```python
from build123d import *

# Parameters (mm, degrees)
SKETCH1_W           = 3
SKETCH1_H           = 6
SKETCH1_W_2         = 16
SKETCH1_H_2         = 3
BOSS_EXTRUDE1_DEPTH = 3


with BuildPart() as part:
    # Sketch1 → Boss-Extrude1 (new body)
    with BuildSketch(Plane(origin=(0, 0, 0), x_dir=(1, 0, 0), z_dir=(0, 1, 0))):
        Polygon((60.5, 0), (60.5, 48), (36, 48), (20, 48), (0, 48), (0, 41), (0, 35), (0, 13), (0, 7), (0, 0), (20, 0), (36, 0), align=None)
        Polygon((85, 48), (60.5, 48), (60.5, 0), (85, 0), (101, 0), (121, 0), (121, 7), (121, 13), (121, 35), (121, 41), (121, 48), (101, 48), align=None)
        with Locations((-1.5, 10)):
            Rectangle(SKETCH1_W, SKETCH1_H)
        with Locations((28, -1.5)):
            Rectangle(SKETCH1_W_2, SKETCH1_H_2)
        with Locations((93, -1.5)):
            Rectangle(SKETCH1_W_2, SKETCH1_H_2)
        with Locations((122.5, 38)):
            Rectangle(SKETCH1_W, SKETCH1_H)
        with Locations((122.5, 10)):
            Rectangle(SKETCH1_W, SKETCH1_H)
        with Locations((-1.5, 38)):
            Rectangle(SKETCH1_W, SKETCH1_H)
        with Locations((28, 49.5)):
            Rectangle(SKETCH1_W_2, SKETCH1_H_2)
        with Locations((93, 49.5)):
            Rectangle(SKETCH1_W_2, SKETCH1_H_2)
    extrude(amount=BOSS_EXTRUDE1_DEPTH)


solid = part.part
```
Can you work these out from the model? Positions are in its coordinate system, mm. A direction names the side the tool comes from. Coordinates: 2 decimals unless noted, no trailing zeros. Write each loop counter-clockwise with the first axis right and the second up, starting at its lowest first coordinate (ties: lowest second). Pieces come first, ordered by that corner, then holes. Notation, with made-up numbers: (11.25, -8.75) - (55.25, -8.75) arc R15 ccw to (55.25, 6.25) - close; hole circle Ø2 at (5.5, 62.5). An arc over 180 degrees is marked (long way). Return JSON: item names as keys, results as strings.
Q1. Thinking about a two-plate mould opening in X: for faces 6 (the flat face through (28, 1, 3)), 7 (the flat face through (61, 1, -48)), 8 (the flat face through (101, 1, 2)), which applies, +X half, -X half, draft (parallel to the pull), parting line (faces both ways), or undercut?
Computed values:
{"face 6": "draft", "face 7": "undercut", "face 8": "+X half"}
Q2. On a 3-axis mill with a long thin cutter (end or side, diameter ignored), from which of +Z, -Z, +X, -X, +Y, -Y can I reach the whole of each face in a straight line? I mean faces 1 (the flat face through (10, 1, 0)), 2 (the flat face through (121, 1, -3)), 3 (the flat face through (60, 1, 0)), 4 (the flat face through (121, 1, -24)), 5 (the flat face through (36, 1, -49)). Say none if no direction works.
Computed values:
{"face 1": "+Z, -X, +Y, -Y", "face 2": "+Z, +X, +Y, -Y", "face 3": "+Z, +Y, -Y", "face 4": "+X, +Y, -Y", "face 5": "-Z, +Y, -Y"}
Q3. If we section it at A-A (x = 113.5): Please give me the cut outline in (y, z).
Computed values:
{"outline": "(0, -48) - (3, -48) - (3, 0) - (0, 0) - close"}
Q4. Please list where these lines run through material, in increasing order: L1, parallel to Z at x = 10.5, y = 1.85; L2, parallel to X at y = 1.25, z = -42.5. Write a range as from..to.
Computed values:
{"L1": "z = -48..0", "L2": "x = 0..121"}
Q5. I'm going to push flat-ended pins straight in: pin 1 Ø0.9 at (x, y) = (9, 2) entering from -Z; pin 2 Ø1.5 at (y, z) = (1.5, -2) entering from +X; pin 3 Ø1.5 at (x, y) = (122.5, 1) entering from +Z. Where does each tip first touch, or does it pass through?
Computed values:
{"pin 1": "stops at z = -48", "pin 2": "stops at x = 121", "pin 3": "stops at z = -7"}
Q6. If we section it at B-B (z = -3.5): Please give me the cut outline in (x, y), then the cut area to 3 significant figures.
Computed values:
{"outline": "(0, 0) - (121, 0) - (121, 3) - (0, 3) - close", "area": "363 mm2"}
